The listing builds one solid part. Answer for the finished solid, in the listing's coordinates (mm). A direction names the side the tool comes from. Round coordinates to 2 decimals unless told otherwise and drop trailing zeros. Order: outer loops, then holes, each group sorted by start corner. A loop starts at its lowest first (then second) coordinate and runs counter-clockwise, first axis right, second up. Notation, with made-up numbers: M 86,53.5 L 98,53.5 A23 ccw 98,65.5 Z; hole C 24,-34.5 d8. An arc over 180 degrees is marked long. Put each result on its own line as item: value. Start each with the question number.
1. The part is cut by section D-D (y = 23.5). Give the vertices of the cut face in (x, z).
2. The part is cut by section B-B (y = 0). Give the vertices of the cut face in (x, z) (1 decimal), then the cut area to 3 significant figures.
3. Each of these flat-tipped pins is pushed along its axis until it touches: pin 1 Ø3 at (x, z) = (14, 2) entering from +Y; pin 2 Ø3 at (x, z) = (-21.5, 1) entering from +Y; pin 3 Ø2.5 at (x, z) = (-46.5, 2.5) entering from +Y. Where does it stop, or does it pass through?
4. The mould has two halves that part along X. Classify faces 1 (the face through (66.674, -0.167, 3.913)), 2 (the face through (-44.04, -22.93, 3.91)), 3 (the face through (60.45, 0.14, 3.91)): +X half, -X half, draft (parallel to the pull), parting line (faces both ways), or undercut.
5. The part is cut by section C-C (z = 5.5). Give the vertices of the cut face in (x, y) (3 decimals).
6. The part is cut by section A-A (x = 0). Give the vertices of the cut face in (y, z).
7. Which of the six approach directions +Z, -Z, +X, -X, +Y, -Y give full straight-line access (tool end or side, diameter ignored) to faces 4 (the face through (44.04, 22.93, 3.91)), 5 (the face through (49, 6.477, 4))?
8. Consider line 1 (X direction, y = 4.5, z = 7.25); line 2 (X direction, y = -1.5, z = 5); line 3 (Y direction, x = 24.5, z = 7.75). Determine where each line is inside the solid, lowest interval first.
from build123d import *

# Parameters (mm, degrees)
F0_R     = 29.21
F1_DEPTH = 7.9375


# Not quite as in the source:
# - a length typed as a fraction of an inch, garbled in the dataset ("3 / 203.2 mm" for 3/8 in), is restored


with BuildPart() as f1:
    # F0 (on Top) → F1 (new body)
    with BuildSketch(Plane.XY):
        with BuildLine():
            Line((-61.4455882353, -10.2703608222), (-26.1470588235, -35.9462628778))
            ThreePointArc((-26.1470588235, -35.9462628778), (0, -44.45), (26.1470588235, -35.9462628778))
            Line((26.1470588235, -35.9462628778), (61.4455882353, -10.2703608222))
            ThreePointArc((61.4455882353, -10.2703608222), (66.675, 0), (61.4455882353, 10.2703608222))
            Line((61.4455882353, 10.2703608222), (26.1470588235, 35.9462628778))
            ThreePointArc((26.1470588235, 35.9462628778), (0, 44.45), (-26.1470588235, 35.9462628778))
            Line((-26.1470588235, 35.9462628778), (-61.4455882353, 10.2703608222))
            ThreePointArc((-61.4455882353, 10.2703608222), (-66.675, 0), (-61.4455882353, -10.2703608222))
        make_face()
        with BuildLine():
            ThreePointArc((-44.069, 6.477), (-37.592, 0), (-44.069, -6.477))
            Line((-44.069, -6.477), (-53.975, -6.477))
            ThreePointArc((-53.975, -6.477), (-60.452, 0), (-53.975, 6.477))
            Line((-53.975, 6.477), (-44.069, 6.477))
        make_face(mode=Mode.SUBTRACT)
        Circle(F0_R, mode=Mode.SUBTRACT)
        with BuildLine():
            ThreePointArc((44.069, -6.477), (37.592, 0), (44.069, 6.477))
            Line((44.069, 6.477), (53.975, 6.477))
            ThreePointArc((53.975, 6.477), (60.452, 0), (53.975, -6.477))
            Line((53.975, -6.477), (44.069, -6.477))
        make_face(mode=Mode.SUBTRACT)
    extrude(amount=F1_DEPTH)


solid = f1.part
Resolved:
1. outline: M -43.26,0 L -17.35,0 L -17.35,7.94 L -43.26,7.94 Z; M 17.35,0 L 43.26,0 L 43.26,7.94 L 17.35,7.94 Z
2. outline: M -66.7,0 L -60.5,0 L -60.5,7.9 L -66.7,7.9 Z; M -37.6,0 L -29.2,0 L -29.2,7.9 L -37.6,7.9 Z; M 29.2,0 L 37.6,0 L 37.6,7.9 L 29.2,7.9 Z; M 60.5,0 L 66.7,0 L 66.7,7.9 L 60.5,7.9 Z
2. area: 232 mm2
3. pin 1: y = 42.66
3. pin 2: y = 39.7
3. pin 3: y = 22.05
4. face 1: +X half
4. face 2: -X half
4. face 3: undercut
5. outline: M -61.446,-10.27 L -26.147,-35.946 A44.45 ccw 26.147,-35.946 L 61.446,-10.27 A12.7 ccw 61.446,10.27 L 26.147,35.946 A44.45 ccw -26.147,35.946 L -61.446,10.27 A12.7 ccw Z; hole M -53.975,-6.477 L -44.069,-6.477 A6.477 ccw -44.069,6.477 L -53.975,6.477 A6.477 ccw Z; hole C 0,0 d58.42; hole M 44.069,-6.477 L 53.975,-6.477 A6.477 ccw 53.975,6.477 L 44.069,6.477 A6.477 ccw Z
6. outline: M -44.45,0 L -29.21,0 L -29.21,7.94 L -44.45,7.94 Z; M 29.21,0 L 44.45,0 L 44.45,7.94 L 29.21,7.94 Z
7. face 4: +Z, -Z, +X, +Y
7. face 5: +Z, -Z
8. line 1: -65.85 to -58.63, -39.41 to -28.86, 28.86 to 39.41, 58.63 to 65.85
8. line 2: -66.59 to -60.28, -37.77 to -29.17, 29.17 to 37.77, 60.28 to 66.59
8. line 3: -37.09 to -15.91, 15.91 to 37.09
